Read the model definition and answer for the solid it produces. Units are mm, in the model's axes. A direction names the side the tool comes from. Coordinates: 2 decimals unless noted, no trailing zeros. Loops run counter-clockwise (first coordinate to the right, second up) from the corner with the lowest first, then second, coordinate; pieces in that order, holes last. Notation, with made-up numbers: (45, -1) - (103, -1) arc R15 ccw to (103, 18) - close; hole circle Ø5 at (3, 41.5). An arc over 180 degrees is marked (long way). Use CSV: the item, a comma, the result in double quotes.
```python
from build123d import *

# Parameters (mm, degrees)
F0_W      = 30
F0_H      = 30
F1_DEPTH  = 20
F3_DEPTH  = 30.001
F8_DEPTH  = 3
F9_DEPTH  = 7.0511256289
F10_R     = 1.25
F11_DEPTH = 8
F12_DEPTH = 7.0511257289
F14_R     = 2.25
F15_DEPTH = 2.9431098966
F16_DEPTH = 7.1080158323


with BuildPart() as f1:
    # F0 (on Front) → F1 (new body)
    with BuildSketch(Plane.XZ):
        with Locations((15, 15)):
            Rectangle(F0_W, F0_H)
    extrude(amount=F1_DEPTH)

    # F2 (on face) → F3 (cut, through all)
    with BuildSketch(Plane.XY.offset(30)):
        with BuildLine():
            Line((0, -20), (30, -20))
            ThreePointArc((30, -20), (15, -11.9498743711), (0, -20))
        make_face()
    extrude(amount=-F3_DEPTH, mode=Mode.SUBTRACT)

    # F7 (on offset) → F8 (cut)
    with BuildSketch(Plane.XZ.offset(12.9498743711)):
        Polygon((17.5, 17.5), (15, 17.5), (12.5, 17.5), (12.5, 16.5), (12.5, 13.5), (12.5, 12.5), (17.5, 12.5), (17.5, 15), align=None)
        Polygon((12.5, 13.5), (12.5, 16.5), (7.5, 16.5), (7.5, 15), (7.5, 13.5), align=None)
    extrude(amount=-F8_DEPTH, mode=Mode.SUBTRACT)

    # F7 (on offset) → F9 (cut, through all)
    with BuildSketch(Plane.XZ.offset(12.9498743711)):
        Polygon((17.5, 17.5), (15, 17.5), (12.5, 17.5), (12.5, 16.5), (12.5, 13.5), (12.5, 12.5), (17.5, 12.5), (17.5, 15), align=None)
        Polygon((12.5, 13.5), (12.5, 16.5), (7.5, 16.5), (7.5, 15), (7.5, 13.5), align=None)
    extrude(amount=F9_DEPTH, mode=Mode.SUBTRACT)

    # F10 (on offset) → F11 (cut)
    with BuildSketch(Plane.XZ.offset(12.9498743711)):
        with Locations((8.5, 17.5)):
            Circle(F10_R)
        with Locations((8.5, 12.5)):
            Circle(F10_R)
    extrude(amount=-F11_DEPTH, mode=Mode.SUBTRACT)

    # F10 (on offset) → F12 (cut, through all)
    with BuildSketch(Plane.XZ.offset(12.9498743711)):
        with Locations((8.5, 17.5)):
            Circle(F10_R)
        with Locations((8.5, 12.5)):
            Circle(F10_R)
    extrude(amount=F12_DEPTH, mode=Mode.SUBTRACT)

    # F14 (on plane+point) → F15 (cut, through all)
    with BuildSketch(Plane.XZ.offset(12.8929842677)):
        with Locations((8.5, 17.5)):
            Circle(F14_R)
        with Locations((8.5, 12.5)):
            Circle(F14_R)
    extrude(amount=-F15_DEPTH, mode=Mode.SUBTRACT)

    # F14 (on plane+point) → F16 (cut, through all)
    with BuildSketch(Plane.XZ.offset(12.8929842677)):
        with Locations((8.5, 17.5)):
            Circle(F14_R)
        with Locations((8.5, 12.5)):
            Circle(F14_R)
    extrude(amount=F16_DEPTH, mode=Mode.SUBTRACT)


solid = f1.part
```
Q1. The part is cut by section C-C on z = 26. Determine the outline of the cut face in (x, y), and give its area (3 significant figures).
Reported:
outline,"(0, -20) arc R18 cw to (30, -20) - (30, 0) - (0, 0) - close"
area,"430 mm²"
Q2. The part is cut by section A-A on y = -11.5. Determine the outline of the cut face in (x, z).
Reported:
outline,"(0, 0) - (30, 0) - (30, 30) - (0, 30) - close; hole (7.5, 14.52) arc R2.25 ccw (long way) to (10.52, 13.5) - (12.5, 13.5) - (12.5, 12.5) - (17.5, 12.5) - (17.5, 17.5) - (12.5, 17.5) - (12.5, 16.5) - (10.52, 16.5) arc R2.25 ccw (long way) to (7.5, 15.48) - close"
Q3. The part is cut by section B-B on x = 8.5. Determine the outline of the cut face in (y, z).
Reported:
outline,"(-13.16, 0) - (0, 0) - (0, 30) - (-13.16, 30) - (-13.16, 19.75) - (-9.95, 19.75) - (-9.95, 18.75) - (-4.95, 18.75) - (-4.95, 16.25) - (-9.95, 16.25) - (-9.95, 13.75) - (-4.95, 13.75) - (-4.95, 11.25) - (-9.95, 11.25) - (-9.95, 10.25) - (-13.16, 10.25) - close"
Q4. Given P1, Ø2, axis at x = 8.5, z = 12.5, coming from the +Y side; P2, Ø5, axis at x = 16, y = -15.5, coming from the -Z side; P3, Ø1.2, axis at x = 9, z = 12.5, coming from the -Y side; P4, Ø2, axis at x = 9, z = 18, coming from the -Y side, each flat-ended and moving along its own axis, determine where each tip first touches the part or whether it passes through.
Reported:
P1,"stops at y = 0"
P2,"passes through"
P3,"stops at y = -4.95"
P4,"stops at y = -9.95"
Q5. For a pull along Z with two mould halves and no side action, classify faces 1 (the face through (30, -10, 15)), 2 (the face through (15, -8, 0)), 3 (the face through (7.25, -7.48, 17.55)), 4 (the face through (15, -8, 30)) as +Z half, -Z half, draft (parallel to the pull), parting line (faces both ways), or undercut.
Reported:
face 1,"draft"
face 2,"-Z half"
face 3,"undercut"
face 4,"+Z half"
Q6. A tool of negligible diameter and unlimited length cuts with its end or side. For faces 5 (the face through (8, -4.95, 13)), 6 (the face through (0, -10, 15)), from which of +Z, -Z, +X, -X, +Y, -Y can it reach the whole face along a straight path? Write none if from no direction.
Reported:
face 5,"-Y"
face 6,"+Z, -Z, -X, +Y, -Y"
Q7. Find the intervals of material crossed by probe 1 along Z at (x, y) = (8.5, -7.5); probe 2 along Z at (x, y) = (8.5, -11.3); probe 3 along X at (y, z) = (-6.05, 12.5), in increasing order. Write a range as [from, to].
Reported:
probe 1,"z = [0, 11.25], [13.75, 16.25], [18.75, 30]"
probe 2,"z = [0, 10.25], [19.75, 30]"
probe 3,"x = [0, 7.25], [9.75, 30]"
Q8. The part is cut by section D-D on x = 16.5. Determine the outline of the cut face in (y, z).
Reported:
outline,"(-12.01, 0) - (0, 0) - (0, 30) - (-12.01, 30) - (-12.01, 17.5) - (-9.95, 17.5) - (-9.95, 12.5) - (-12.01, 12.5) - close"
